```python
from build123d import *

# Parameters (mm, degrees)
ESBO_O1_W                = 80
ESBO_O1_H                = 60
ESBO_O1_R                = 6.25
RESSALTO_EXTRUS_O1_DEPTH = 6
CHANFRO1_SIZE            = 3


with BuildPart() as part:
    # Esboço1 → Ressalto-extrusão1 (new body)
    with BuildSketch(Plane(origin=(0, 0, 0), x_dir=(0, 0, -1), z_dir=(1, 0, 0))):
        with Locations((40, 30)):
            Rectangle(ESBO_O1_W, ESBO_O1_H)
        with Locations((12, 10.327729246)):
            Circle(ESBO_O1_R, mode=Mode.SUBTRACT)
        with Locations((12, 47.872237221)):
            Circle(ESBO_O1_R, mode=Mode.SUBTRACT)
        with Locations((52, 47.872237221)):
            Circle(ESBO_O1_R, mode=Mode.SUBTRACT)
        with Locations((52, 10.327729246)):
            Circle(ESBO_O1_R, mode=Mode.SUBTRACT)
    extrude(amount=RESSALTO_EXTRUS_O1_DEPTH)

    # Chanfro1
    chanfro1_edges = [part.edges().sort_by_distance(p)[0] for p in [
        (6, 10.327729246, -5.75),
        (6, 47.872237221, -5.75),
        (6, 47.872237221, -45.75),
        (6, 10.327729246, -45.75),
    ]]
    chamfer(chanfro1_edges, length=CHANFRO1_SIZE)


solid = part.part
```
Design review of the part built by this model. Coordinates are the model's own, in mm. Coordinates: 2 decimals unless noted, no trailing zeros. Write each loop counter-clockwise with the first axis right and the second up, starting at its lowest first coordinate (ties: lowest second). Pieces come first, ordered by that corner, then holes.
1) To check wall thickness, follow L1, parallel to Y at x = 1.6, z = -52; L2, parallel to Y at x = 5.6, z = -56.5; L3, parallel to Z at x = 0.8, y = 51. State the ranges of each line that lie inside material, in increasing order.
2) Insertion check: pin 1 (10 mm diameter, centred on y = 47.87, z = -52, fed in from +X); pin 2 (3 mm diameter, centred on x = 3.5, z = -29.5, fed in from -Y). Each pin has a flat end and moves straight along its axis. Give the tip position at first contact, or say it passes through.
3) Add section A-A (z = -12). Write out the cut boundary in (x, y).
4) Mouldability with a two-part tool opening along Y and no side actions: class faces 1 (the flat face through (0, 30, -39)), 2 (the conical face through (3.19, 4.04, -50.6)), 3 (the flat face through (3, 60, -39)), 4 (the cylindrical face through (1.48, 53.14, -55.36)) as +Y half, -Y half, draft (parallel to the pull), parting line (faces both ways), or undercut.
5) Add section B-B (x = 1.9). Write out the cut boundary in (y, z).
6) Add section C-C (y = 12.5). State how many separate pieces and enclosed holes the cut face has, plus the area to 3 significant figures.
Check result:
1. L1: y = 0 to 4.08, 16.58 to 41.62, 54.12 to 60
1. L2: y = 0 to 2.71, 17.95 to 40.25, 55.49 to 60
1. L3: z = -80 to -57.41, -46.59 to -17.41, -6.59 to 0
2. pin 1: passes through
2. pin 2: stops at y = 0
3. outline: (0, 0) - (6, 0) - (6, 1.08) - (3, 4.08) - (0, 4.08) - close; (0, 16.58) - (3, 16.58) - (6, 19.58) - (6, 38.62) - (3, 41.62) - (0, 41.62) - close; (0, 54.12) - (3, 54.12) - (6, 57.12) - (6, 60) - (0, 60) - close
4. face 1: draft
4. face 2: undercut
4. face 3: +Y half
4. face 4: undercut
5. outline: (0, -80) - (60, -80) - (60, 0) - (0, 0) - close; hole circle Ø12.5 at (10.33, -52); hole circle Ø12.5 at (10.33, -12); hole circle Ø12.5 at (47.87, -52); hole circle Ø12.5 at (47.87, -12)
6. separate pieces: 3
6. enclosed holes: 0
6. area: 320 mm2
